```python
from build123d import *

# Parameters (mm, degrees)
SKETCH1_W                                  = 150
SKETCH1_H                                  = 60
BOSS_EXTRUDE1_DEPTH                        = 10
CUT_EXTRUDE1_DEPTH                         = 84.216584885
CUT_EXTRUDE1_DEPTH_BACK                    = 84.216584885
SKETCH2_W                                  = 130
SKETCH2_H                                  = 10
FILLET1_R                                  = 5
SKETCH4_R                                  = 1.7
CUT_EXTRUDE3_DEPTH                         = 144.527000944
CUT_EXTRUDE4_DEPTH                         = 3
MIRROR1_AT_THE_SECOND_PLANE_COPY_1_SKETC_R = 1.7
MIRROR1_AT_THE_SECOND_PLANE_COPY_1_DEPTH   = 144.527000944
MIRROR1_AT_THE_SECOND_PLANE_COPY_2_DEPTH   = 3
MIRROR2_COPY_1_SKETCH_R                    = 1.7
MIRROR2_COPY_1_DEPTH                       = 144.527000944
MIRROR2_COPY_2_DEPTH                       = 3
MIRROR2_COPY_3_SKETCH_R                    = 1.7
MIRROR2_COPY_3_DEPTH                       = 144.527000944
MIRROR2_COPY_4_DEPTH                       = 3
MIRROR2_COPY_5_SKETCH_R                    = 1.7
MIRROR2_COPY_5_DEPTH                       = 144.527000944
MIRROR2_COPY_6_DEPTH                       = 3
MIRROR2_COPY_7_SKETCH_R                    = 1.7
MIRROR2_COPY_7_DEPTH                       = 144.527000944
SKETCH6_R                                  = 12.5
CUT_EXTRUDE5_DEPTH                         = 84.216584885


with BuildPart() as part:
    # Sketch1 → Boss-Extrude1 (new, symmetric)
    with BuildSketch(Plane.XY):
        Rectangle(SKETCH1_W, SKETCH1_H)
    extrude(amount=BOSS_EXTRUDE1_DEPTH, both=True)

    # Sketch2 → Cut-Extrude1 (cut, two sides: drawn at the far end of the back side and taken through both)
    with BuildSketch(Plane.XY.offset(10).offset(-CUT_EXTRUDE1_DEPTH_BACK)):
        with Locations((0, -25)):
            Rectangle(SKETCH2_W, SKETCH2_H)
        with Locations((0, 25)):
            Rectangle(SKETCH2_W, SKETCH2_H)
    extrude(amount=CUT_EXTRUDE1_DEPTH + CUT_EXTRUDE1_DEPTH_BACK, mode=Mode.SUBTRACT)

    # Fillet1
    fillet1_edges = [part.edges().sort_by_distance(p)[0] for p in [
        (70, -30, -10),
        (-70, 30, -10),
        (-70, -30, 10),
        (-70, 30, 10),
        (70, -30, 10),
        (-70, -30, -10),
        (70, 30, -10),
        (70, 30, 10),
    ]]
    fillet(fillet1_edges, radius=FILLET1_R)

    # Sketch4 → Cut-Extrude3 (cut, symmetric)
    with BuildSketch(Plane.ZY.offset(-65)):
        with Locations((-5, 25)):
            Circle(SKETCH4_R)
    cut_extrude3 = extrude(amount=CUT_EXTRUDE3_DEPTH, both=True, mode=Mode.SUBTRACT)

    # Sketch5 → Cut-Extrude4 (cut)
    with BuildSketch(Plane.ZY.offset(-65)):
        Polygon((-8.464101615, 25), (-6.732050808, 22), (-3.267949192, 22), (-1.535898385, 25), (-3.267949192, 28), (-6.732050808, 28), align=None)
    cut_extrude4 = extrude(amount=-CUT_EXTRUDE4_DEPTH, mode=Mode.SUBTRACT)

    # Mirror1: Cut-Extrude3, Cut-Extrude4 across plane
    add(cut_extrude3.mirror(Plane(origin=(0, 0, 0), x_dir=(0, 0, 1), z_dir=(1, 0, 0))), mode=Mode.SUBTRACT)
    add(cut_extrude4.mirror(Plane(origin=(0, 0, 0), x_dir=(0, 0, 1), z_dir=(1, 0, 0))), mode=Mode.SUBTRACT)

    # Mirror1 at the second plane: Cut-Extrude3, Cut-Extrude4 across plane
    add(cut_extrude3.mirror(Plane.XY), mode=Mode.SUBTRACT)
    add(cut_extrude4.mirror(Plane.XY), mode=Mode.SUBTRACT)

    # Mirror1 at the second plane copy 1 sketc → Mirror1 at the second plane copy 1 (cut, symmetric)
    with BuildSketch(Plane(origin=(-65, 0, 0), x_dir=(0, 0, -1), z_dir=(1, 0, 0))):
        with Locations((-5, 25)):
            Circle(MIRROR1_AT_THE_SECOND_PLANE_COPY_1_SKETC_R)
    extrude(amount=MIRROR1_AT_THE_SECOND_PLANE_COPY_1_DEPTH, both=True, mode=Mode.SUBTRACT)

    # Mirror1 at the second plane copy 2 sketc → Mirror1 at the second plane copy 2 (cut)
    with BuildSketch(Plane(origin=(-65, 0, 0), x_dir=(0, 0, -1), z_dir=(1, 0, 0))):
        Polygon((-8.464101615, 25), (-6.732050808, 22), (-3.267949192, 22), (-1.535898385, 25), (-3.267949192, 28), (-6.732050808, 28), align=None)
    extrude(amount=-MIRROR1_AT_THE_SECOND_PLANE_COPY_2_DEPTH, mode=Mode.SUBTRACT)

    # Mirror2: Cut-Extrude4 across plane
    add(cut_extrude4.mirror(Plane.ZX), mode=Mode.SUBTRACT)

    # Mirror2 copy 1 sketch → Mirror2 copy 1 (cut, symmetric)
    with BuildSketch(Plane(origin=(-65, 0, 0), x_dir=(0, 0, 1), z_dir=(1, 0, 0))):
        with Locations((-5, 25)):
            Circle(MIRROR2_COPY_1_SKETCH_R)
    extrude(amount=MIRROR2_COPY_1_DEPTH, both=True, mode=Mode.SUBTRACT)

    # Mirror2 copy 2 sketch → Mirror2 copy 2 (cut)
    with BuildSketch(Plane(origin=(-65, 0, 0), x_dir=(0, 0, 1), z_dir=(1, 0, 0))):
        Polygon((-8.464101615, 25), (-6.732050808, 22), (-3.267949192, 22), (-1.535898385, 25), (-3.267949192, 28), (-6.732050808, 28), align=None)
    extrude(amount=-MIRROR2_COPY_2_DEPTH, mode=Mode.SUBTRACT)

    # Mirror2 copy 3 sketch → Mirror2 copy 3 (cut, symmetric)
    with BuildSketch(Plane(origin=(65, 0, 0), x_dir=(0, 0, -1), z_dir=(-1, 0, 0))):
        with Locations((-5, 25)):
            Circle(MIRROR2_COPY_3_SKETCH_R)
    extrude(amount=MIRROR2_COPY_3_DEPTH, both=True, mode=Mode.SUBTRACT)

    # Mirror2 copy 4 sketch → Mirror2 copy 4 (cut)
    with BuildSketch(Plane(origin=(65, 0, 0), x_dir=(0, 0, -1), z_dir=(-1, 0, 0))):
        Polygon((-8.464101615, 25), (-6.732050808, 22), (-3.267949192, 22), (-1.535898385, 25), (-3.267949192, 28), (-6.732050808, 28), align=None)
    extrude(amount=-MIRROR2_COPY_4_DEPTH, mode=Mode.SUBTRACT)

    # Mirror2 copy 5 sketch → Mirror2 copy 5 (cut, symmetric)
    with BuildSketch(Plane(origin=(-65, 0, 0), x_dir=(0, 0, -1), z_dir=(1, 0, 0))):
        with Locations((-5, -25)):
            Circle(MIRROR2_COPY_5_SKETCH_R)
    extrude(amount=MIRROR2_COPY_5_DEPTH, both=True, mode=Mode.SUBTRACT)

    # Mirror2 copy 6 sketch → Mirror2 copy 6 (cut)
    with BuildSketch(Plane(origin=(-65, 0, 0), x_dir=(0, 0, -1), z_dir=(1, 0, 0))):
        Polygon((-8.464101615, -25), (-6.732050808, -22), (-3.267949192, -22), (-1.535898385, -25), (-3.267949192, -28), (-6.732050808, -28), align=None)
    extrude(amount=-MIRROR2_COPY_6_DEPTH, mode=Mode.SUBTRACT)

    # Mirror2 copy 7 sketch → Mirror2 copy 7 (cut, symmetric)
    with BuildSketch(Plane.ZY.offset(-65)):
        with Locations((-5, -25)):
            Circle(MIRROR2_COPY_7_SKETCH_R)
    extrude(amount=MIRROR2_COPY_7_DEPTH, both=True, mode=Mode.SUBTRACT)

    # Sketch6 → Cut-Extrude5 (cut, through all)
    with BuildSketch(Plane(origin=(0, 0, -10), x_dir=(-1, 0, 0), z_dir=(0, 0, -1))):
        Circle(SKETCH6_R)
    extrude(amount=-CUT_EXTRUDE5_DEPTH, mode=Mode.SUBTRACT)


solid = part.part
```
Build history of the part. All positions in model axes, mm. A direction names the side the tool comes from. Coordinates: 2 decimals unless noted, no trailing zeros. Order: outer loops, then holes, each group sorted by start corner. A loop starts at its lowest first (then second) coordinate and runs counter-clockwise, first axis right, second up. Notation, with made-up numbers: M 34,-6 L 48,-6 A18 cw 48,19 Z; hole C -13,21.5 d4. An arc over 180 degrees is marked long. One line per question, with ' | ' between items. Start each with the question number.
1. Flat gauge pins, fed straight in: P1, Ø0.9, axis at x = 66, z = -6, coming from the +Y side; P2, Ø2, axis at x = -33.5, z = -1, coming from the +Y side; P3, Ø2, axis at x = -15, z = -5, coming from the -Y side. Where does each tip first touch, or does it go through?
2. Tool access for faces 5 (the face through (-1, 20, 0)), 6 (the face through (66.5, -23.5, -7.6)): list every direction of +Z, -Z, +X, -X, +Y, -Y with a clear straight run to the whole face (end or side of a thin tool).
3. Mould opens along Y. For faces 1 (the face through (-66.5, -23.5, 2.4)), 2 (the face through (70, -28, 9)), 3 (the face through (66.5, 23.5, -7.6)), 4 (the face through (75, 0, 0)) say: +Y half, -Y half, draft (parallel to the pull), parting line (faces both ways), or undercut.
4. Cut at C-C (y = 8.5). Write the cut outline in (x, z), plus the area to 3 significant figures.
5. Cut at B-B (x = -55.5). Write the cut outline in (y, z), plus the area to 3 significant figures.
6. Wall check: line 1 along Y through (x, z) = (-73.5, -5); line 2 along X through (y, z) = (25, -2.25); line 3 along X through (y, z) = (-22, 1.75). Give the ranges that are in metal, low to high. Write a range as [from, to].
7. Cut at A-A (y = 0). Write the cut outline in (x, z), plus the area to 3 significant figures.
The answers:
1) P1: stops at y = 29.97 | P2: stops at y = 20 | P3: stops at y = -20
2) face 5: +Z, -Z, +Y | face 6: none
3) face 1: undercut | face 2: -Y half | face 3: undercut | face 4: draft
4) outline: M -75,-10 L -9.17,-10 L -9.17,10 L -75,10 Z; M 9.17,-10 L 75,-10 L 75,10 L 9.17,10 Z | area: 2,630 mm2
5) outline: M -20,-10 L 20,-10 L 20,10 L -20,10 Z | area: 800 mm2
6) line 1: y = [-30, -26.7], [-23.3, 23.3], [26.7, 30] | line 2: x = [-75, -68], [68, 75] | line 3: x = [-75, -65], [65, 75]
7) outline: M -75,-10 L -12.5,-10 L -12.5,10 L -75,10 Z; M 12.5,-10 L 75,-10 L 75,10 L 12.5,10 Z | area: 2,500 mm2
